Model file for the job. Use its own axes, mm. Round coordinates to 2 decimals unless told otherwise and drop trailing zeros. Loops run counter-clockwise (first coordinate to the right, second up) from the corner with the lowest first, then second, coordinate; pieces in that order, holes last. Notation, with made-up numbers: M -20.5,45.25 L 32.5,45.25 A18 cw 32.5,74.25 Z; hole C -23,19 d7. An arc over 180 degrees is marked long. Use a Markdown table: item, result. Add a question column.
Q1. Pin check, flat tips, straight feed: pin 1 (2 mm diameter, centred on x = 13, z = 19, fed in from -Y); pin 2 (3 mm diameter, centred on x = -29, y = -15.5, fed in from +Z); pin 3 (1.5 mm diameter, centred on y = -4.5, z = 19, fed in from +X). Stop position of each tip, or through.
Q2. Cut at D-D (x = 13). Give the cut face in (y, z), plus the area to 3 significant figures.
Q3. Cut at A-A (x = -27). Give the cut face in (y, z), plus the area to 3 significant figures.
Q4. Probe line 1 (Y direction, x = -12, z = 19); line 2 (Z direction, x = 8.5, y = -10.5); line 3 (Y direction, x = -6, z = 20.5). List the from-to ranges inside material, lowest first. Write a range as from..to.
Q5. Cut at B-B (y = -8.25). Give the cut face in (x, z).
Q6. Cut at C-C (z = 18). State how many separate pieces and enclosed holes the cut face has, plus the area to 3 significant figures.
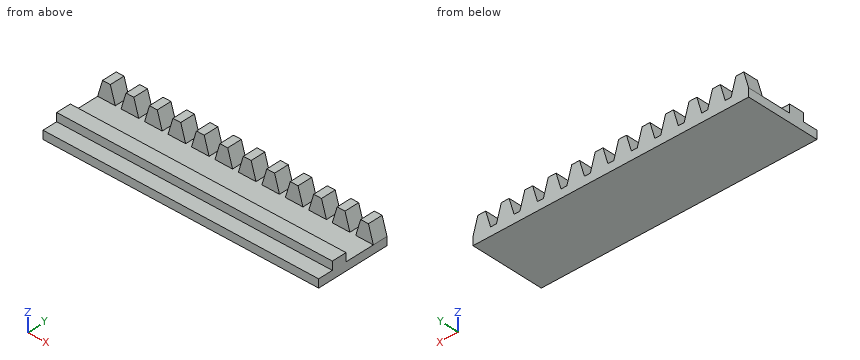
from build123d import *

# Parameters (mm, degrees)
F1_DEPTH = 3.81
F4_DEPTH = 71.628


with BuildPart() as f1:
    # F0 (on Front) → F1 (new body)
    with BuildSketch(Plane.XZ):
        Polygon((-38.4448663006, 16.8945933835), (-38.4448663006, 14.7355933835), (33.1831336994, 14.7355933835), (33.1831336994, 16.8945933835), (28.6111336994, 16.8945933835), (27.0871336994, 16.8945933835), (22.5151336994, 16.8945933835), (20.9911336994, 16.8945933835), (16.4191336994, 16.8945933835), (14.8951336994, 16.8945933835), (10.3231336994, 16.8945933835), (8.7991336994, 16.8945933835), (4.2271336994, 16.8945933835), (2.7031336994, 16.8945933835), (-1.8688663006, 16.8945933835), (-3.3928663006, 16.8945933835), (-7.9648663006, 16.8945933835), (-9.4888663006, 16.8945933835), (-14.0608663006, 16.8945933835), (-15.5848663006, 16.8945933835), (-20.1568663006, 16.8945933835), (-21.6808663006, 16.8945933835), (-26.2528663006, 16.8945933835), (-27.7768663006, 16.8945933835), (-32.3488663006, 16.8945933835), (-33.8728663006, 16.8945933835), align=None)
        Polygon((-37.1748663006, 21.2125933835), (-38.4448663006, 16.8945933835), (-33.8728663006, 16.8945933835), (-35.1428663006, 21.2125933835), align=None)
        Polygon((28.6111336994, 16.8945933835), (33.1831336994, 16.8945933835), (31.9131336994, 21.2125933835), (29.8811336994, 21.2125933835), align=None)
        Polygon((-31.0788663006, 21.2125933835), (-32.3488663006, 16.8945933835), (-27.7768663006, 16.8945933835), (-29.0468663006, 21.2125933835), align=None)
        Polygon((22.5151336994, 16.8945933835), (27.0871336994, 16.8945933835), (25.8171336994, 21.2125933835), (23.7851336994, 21.2125933835), align=None)
        Polygon((-24.9828663006, 21.2125933835), (-26.2528663006, 16.8945933835), (-21.6808663006, 16.8945933835), (-22.9508663006, 21.2125933835), align=None)
        Polygon((16.4191336994, 16.8945933835), (20.9911336994, 16.8945933835), (19.7211336994, 21.2125933835), (17.6891336994, 21.2125933835), align=None)
        Polygon((-18.8868663006, 21.2125933835), (-20.1568663006, 16.8945933835), (-15.5848663006, 16.8945933835), (-16.8548663006, 21.2125933835), align=None)
        Polygon((10.3231336994, 16.8945933835), (14.8951336994, 16.8945933835), (13.6251336994, 21.2125933835), (11.5931336994, 21.2125933835), align=None)
        Polygon((-12.7908663006, 21.2125933835), (-14.0608663006, 16.8945933835), (-9.4888663006, 16.8945933835), (-10.7588663006, 21.2125933835), align=None)
        Polygon((4.2271336994, 16.8945933835), (8.7991336994, 16.8945933835), (7.5291336994, 21.2125933835), (5.4971336994, 21.2125933835), align=None)
        Polygon((-6.6948663006, 21.2125933835), (-7.9648663006, 16.8945933835), (-3.3928663006, 16.8945933835), (-4.6628663006, 21.2125933835), align=None)
        Polygon((-1.8688663006, 16.8945933835), (2.7031336994, 16.8945933835), (1.4331336994, 21.2125933835), (-0.5988663006, 21.2125933835), align=None)
    extrude(amount=F1_DEPTH)

    # F3 (on plane+point) → F4 (join, through all)
    with BuildSketch(Plane.YZ.offset(33.1831336994)):
        Polygon((-19.05, 14.7355933835), (-3.81, 14.7355933835), (-3.81, 16.8945933835), (-11.43, 16.8945933835), (-11.43, 19.0535933835), (-15.24, 19.0535933835), (-15.24, 16.8945933835), (-19.05, 16.8945933835), align=None)
    extrude(amount=-F4_DEPTH)


solid = f1.part
Checked values:
| question | item | result |
|---|---|---|
| 1 | pin 1 | stops at y = -15.24 |
| 1 | pin 2 | stops at z = 19.05 |
| 1 | pin 3 | stops at x = 32.65 |
| 2 | outline | M -19.05,14.74 L 0,14.74 L 0,21.21 L -3.81,21.21 L -3.81,16.89 L -11.43,16.89 L -11.43,19.05 L -15.24,19.05 L -15.24,16.89 L -19.05,16.89 Z |
| 2 | area | 65.8 mm^2 |
| 3 | outline | M -19.05,14.74 L 0,14.74 L 0,16.89 L -11.43,16.89 L -11.43,19.05 L -15.24,19.05 L -15.24,16.89 L -19.05,16.89 Z |
| 3 | area | 49.4 mm^2 |
| 4 | line 1 | y = -15.24..-11.43, -3.81..0 |
| 4 | line 2 | z = 14.74..16.89 |
| 4 | line 3 | y = -3.81..0 |
| 5 | outline | M -38.44,14.74 L 33.18,14.74 L 33.18,16.89 L -38.44,16.89 Z |
| 6 | separate pieces | 13 |
| 6 | enclosed holes | 0 |
| 6 | area | 452 mm^2 |
